Input: dimensioned drawing with shaded views. Units: mm. Origin: part minimum x, y, z. A direction names the side the tool comes from. Give positions to 0.01 mm unless a question says otherwise; leave off trailing zeros. Order: outer loops, then holes, each group sorted by start corner. A loop starts at its lowest first (then second) coordinate and runs counter-clockwise, first axis right, second up.
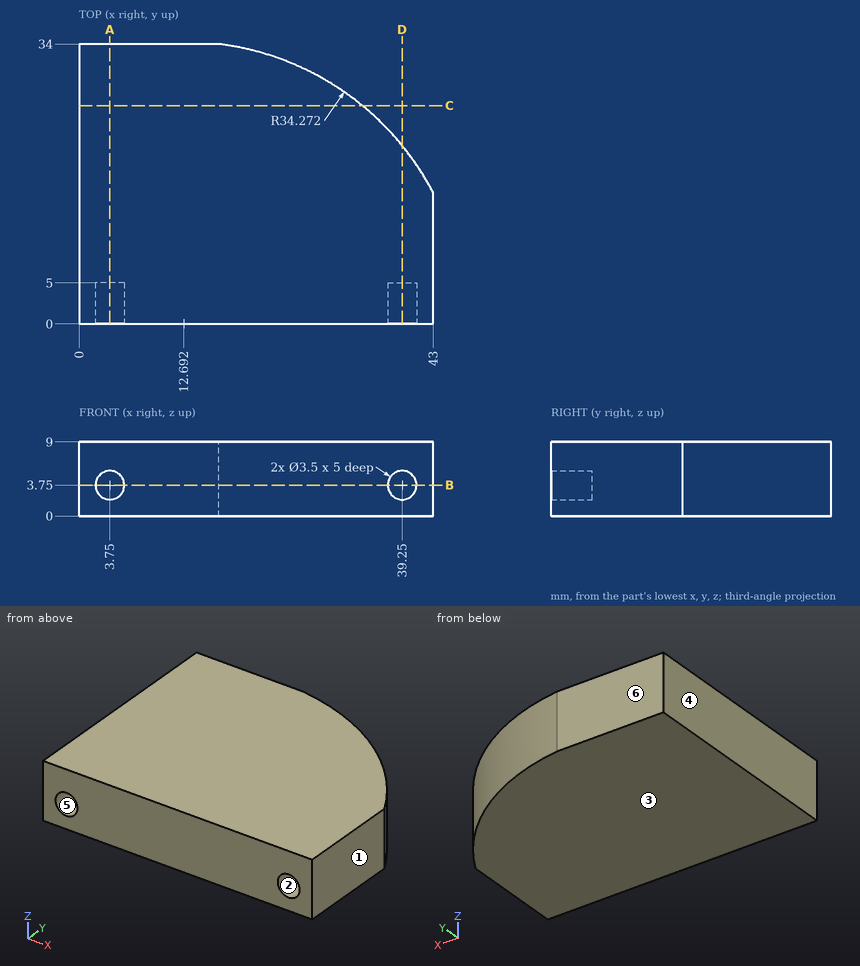
1) Draft query along X for the marked faces 1, 2, 3 and 4. Return one class per face: +X half, -X half, draft (parallel to the pull), parting line (faces both ways), or undercut.
Report:
face 1: +X half
face 2: undercut
face 3: draft
face 4: -X half
2) Pin query (flat end, axial travel): pin 1 (1 mm diameter, centred on x = 39, z = 3, fed in from -Y); pin 2 (5 mm diameter, centred on y = 23, z = 6, fed in from +X). Return the tip coordinate at first contact, or that it passes through.
Report:
pin 1: stops at y = 5
pin 2: stops at x = 40.16
3) Section query B-B, the plane z = 3.75. Return the cut outline in (x, y).
Report:
outline: (0, 0) - (2, 0) - (2, 5) - (5.5, 5) - (5.5, 0) - (37.5, 0) - (37.5, 5) - (41, 5) - (41, 0) - (43, 0) - (43, 16) arc R34.27 ccw to (17, 34) - (0, 34) - close
4) Reachability of the marked faces 5 and 6 from +Z, -Z, +X, -X, +Y, -Y: full face, straight path, thin tool, end or side. Return the list, or none.
Report:
face 5: -Y
face 6: +Z, -Z, +X, -X, +Y
5) Section query A-A, the plane x = 3.75. Return the cut outline in (y, z).
Report:
outline: (0, 0) - (34, 0) - (34, 9) - (0, 9) - (0, 5.5) - (5, 5.5) - (5, 2) - (0, 2) - close
6) Material intervals for L1, parallel to X at y = 1.1, z = 3.75; L2, parallel to X at y = 3, z = 2.5 (1 decimal); L3, parallel to Z at x = 39.25, y = 1.5, sorted ascending.
Report:
L1: x = 0 to 2, 5.5 to 37.5, 41 to 43
L2: x = 0 to 2.5, 5 to 38, 40.5 to 43
L3: z = 0 to 2, 5.5 to 9
7) Section query D-D, the plane x = 39.25. Return the cut outline in (y, z).
Report:
outline: (0, 0) - (21.66, 0) - (21.66, 9) - (0, 9) - (0, 5.5) - (5, 5.5) - (5, 2) - (0, 2) - close
8) Section query C-C, the plane y = 26.5. Return the cut outline in (x, z) (1 decimal).
Report:
outline: (0, 0) - (34.4, 0) - (34.4, 9) - (0, 9) - close
